Design review of the part shown in the three views and the two pictorial views. Dimensions are in mm from the part's minimum x, y and z. A direction names the side the tool comes from. Give positions to 0.01 mm unless a question says otherwise; leave off trailing zeros. Loops run counter-clockwise (first coordinate to the right, second up) from the corner with the lowest first, then second, coordinate; pieces in that order, holes last. Notation, with made-up numbers: (54.25, -25.75) -> (85.25, -25.75) arc R10 ccw to (85.25, -20.75) -> close; hole circle Ø2 at (-6.5, 16). An arc over 180 degrees is marked (long way). Answer as CSV lines item,"result".
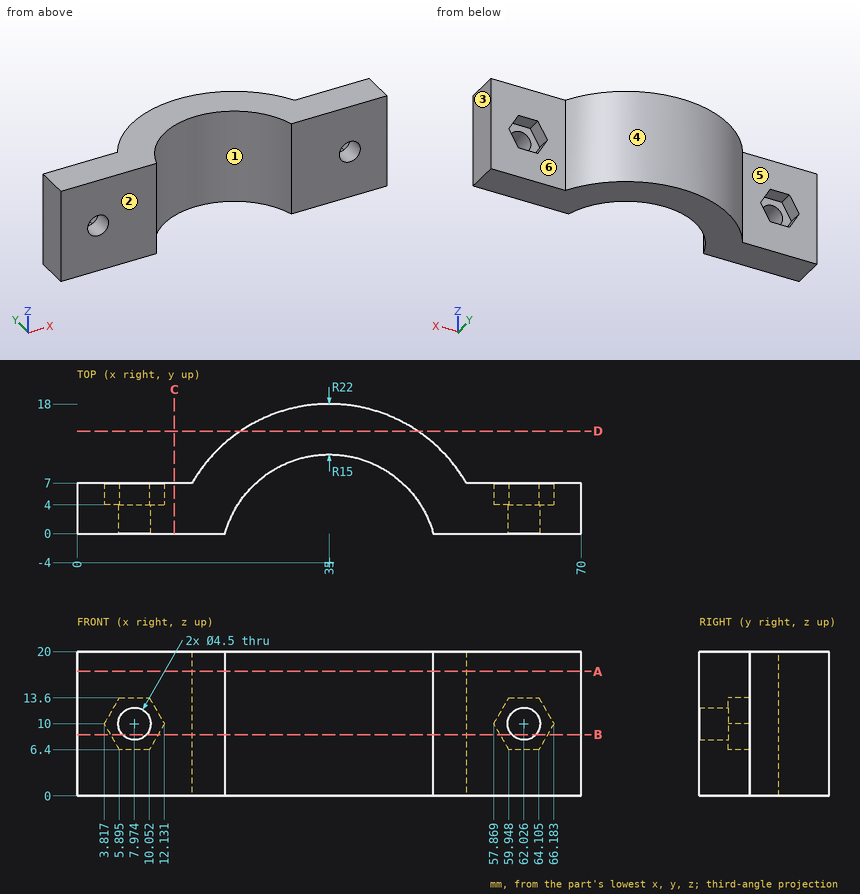
Q1. We need section C-C, the plane x = 13.5. State the section outline as (y, z) points.
Filled sheet:
outline,"(0, 0) -> (7, 0) -> (7, 20) -> (0, 20) -> close"
Q2. Clearance check with flat-ended pins moving along their axes: pin 1 Ø1.5 at (x, z) = (22.5, 13.5) entering from -Y; pin 2 Ø3 at (x, y) = (28, 7) entering from +Z; pin 3 Ø2 at (y, z) = (13.5, 16.5) entering from +X; pin 4 Ø1 at (y, z) = (14.5, 5) entering from -X. State where each tip first meets the part, or that it passes through.
Filled sheet:
pin 1,"stops at y = 3.03"
pin 2,"passes through"
pin 3,"stops at x = 49.55"
pin 4,"stops at x = 22.35"
Q3. To check wall thickness, follow probe 1 along Z at (x, y) = (61, 5.5); probe 2 along Y at (x, z) = (10, 17.5); probe 3 along Y at (x, z) = (59, 11.5). State the ranges of each line that lie inside material, in increasing order. Write a range as from..to.
Filled sheet:
probe 1,"z = 0..6.4, 13.6..20"
probe 2,"y = 0..7"
probe 3,"y = 0..4"
Q4. We need section D-D, the plane y = 14.25. State the section outline as (x, z) points (1 decimal).
Filled sheet:
outline,"(22.7, 0) -> (47.3, 0) -> (47.3, 20) -> (22.7, 20) -> close"
Q5. The part is to be moulded in two halves that separate along X. For the marked faces 1, 2 and 3, say which applies: pulls with the +X half, pulls with the -X half, needs draft (parallel to the pull), parting line crosses it, or undercut.
Filled sheet:
face 1,"undercut"
face 2,"needs draft"
face 3,"pulls with the +X half"
Q6. For the marked faces 4, 5 and 6, list the 3-axis set-ups (+Z, -Z, +X, -X, +Y, -Y) from which the entire face can be reached by the end or side of a thin tool; tool diameter is ignored.
Filled sheet:
face 4,"+Z, -Z, +Y"
face 5,"+Z, -Z, -X, +Y"
face 6,"+Z, -Z, +X, +Y"
Q7. We need section A-A, the plane z = 17.25. State the section outline as (x, y) points.
Filled sheet:
outline,"(0, 0) -> (20.54, 0) arc R15 cw to (49.46, 0) -> (70, 0) -> (70, 7) -> (54.05, 7) arc R22 ccw to (15.95, 7) -> (0, 7) -> close"
Q8. We need section B-B, the plane z = 8.5. State the section outline as (x, y) points (1 decimal).
Filled sheet:
outline,"(0, 0) -> (6.3, 0) -> (6.3, 4) -> (4.7, 4) -> (4.7, 7) -> (0, 7) -> close; (9.7, 0) -> (20.5, 0) arc R15 cw to (49.5, 0) -> (60.3, 0) -> (60.3, 4) -> (58.7, 4) -> (58.7, 7) -> (54.1, 7) arc R22 ccw to (15.9, 7) -> (11.3, 7) -> (11.3, 4) -> (9.7, 4) -> close; (63.7, 0) -> (70, 0) -> (70, 7) -> (65.3, 7) -> (65.3, 4) -> (63.7, 4) -> close"
